For this review, take the finished solid that the model builds, in its own axes (mm). A direction names the side the tool comes from. Coordinates: 2 decimals unless noted, no trailing zeros. Order: outer loops, then holes, each group sorted by start corner. A loop starts at its lowest first (then second) coordinate and runs counter-clockwise, first axis right, second up. Notation, with made-up numbers: M 69,38 L 97,38 A12 cw 97,52 Z; hole C -9,37.5 d7. An arc over 180 degrees is marked long. Use CSV: the item, a comma, the result in double quotes.
```python
from build123d import *

# Parameters (mm, degrees)
SKETCH1_R           = 5
BOSS_EXTRUDE1_DEPTH = 10


with BuildPart() as part:
    # Sketch1 → Boss-Extrude1 (new body)
    with BuildSketch(Plane(origin=(0, 0, 0), x_dir=(1, 0, 0), z_dir=(0, 1, 0))):
        with BuildLine():
            ThreePointArc((7.500789876, 99.718293965), (6.250885533, 99.804440934), (5, 99.874921777))
            Line((5, 99.874921777), (5, 57.735026919))
            ThreePointArc((5, 57.735026919), (0, 52.735026919), (-5, 57.735026919))
            Line((-5, 57.735026919), (-5, 99.874921777))
            ThreePointArc((-5, 99.874921777), (-6.250885533, 99.804440934), (-7.500789876, 99.718293965))
            ThreePointArc((-7.500789876, 99.718293965), (-32.617513459, 56.495190528), (-82.608180857, 56.355021564))
            ThreePointArc((-82.608180857, 56.355021564), (-83.307738492, 55.315646135), (-83.99421946, 54.267587908))
            Line((-83.99421946, 54.267587908), (-47.5, 33.197640478))
            ThreePointArc((-47.5, 33.197640478), (-45.669872981, 26.367513459), (-52.5, 24.537386441))
            Line((-52.5, 24.537386441), (-88.99421946, 45.60733387))
            ThreePointArc((-88.99421946, 45.60733387), (-89.558624026, 44.488794799), (-90.108970734, 43.363272401))
            ThreePointArc((-90.108970734, 43.363272401), (-65.235026919, 0), (-90.108970734, -43.363272401))
            ThreePointArc((-90.108970734, -43.363272401), (-89.558624026, -44.488794799), (-88.99421946, -45.60733387))
            Line((-88.99421946, -45.60733387), (-52.5, -24.537386441))
            ThreePointArc((-52.5, -24.537386441), (-45.669872981, -26.367513459), (-47.5, -33.197640478))
            Line((-47.5, -33.197640478), (-83.99421946, -54.267587908))
            ThreePointArc((-83.99421946, -54.267587908), (-83.307738492, -55.315646135), (-82.608180857, -56.355021564))
            ThreePointArc((-82.608180857, -56.355021564), (-32.617513459, -56.495190528), (-7.500789876, -99.718293965))
            ThreePointArc((-7.500789876, -99.718293965), (-6.250885533, -99.804440934), (-5, -99.874921777))
            Line((-5, -99.874921777), (-5, -57.735026919))
            ThreePointArc((-5, -57.735026919), (0, -52.735026919), (5, -57.735026919))
            Line((5, -57.735026919), (5, -99.874921777))
            ThreePointArc((5, -99.874921777), (6.250885533, -99.804440934), (7.500789876, -99.718293965))
            ThreePointArc((7.500789876, -99.718293965), (32.617513459, -56.495190528), (82.608180857, -56.355021564))
            ThreePointArc((82.608180857, -56.355021564), (83.307738492, -55.315646135), (83.99421946, -54.267587908))
            Line((83.99421946, -54.267587908), (47.5, -33.197640478))
            ThreePointArc((47.5, -33.197640478), (45.669872981, -26.367513459), (52.5, -24.537386441))
            Line((52.5, -24.537386441), (88.99421946, -45.60733387))
            ThreePointArc((88.99421946, -45.60733387), (89.558624026, -44.488794799), (90.108970734, -43.363272401))
            ThreePointArc((90.108970734, -43.363272401), (65.235026919, 0), (90.108970734, 43.363272401))
            ThreePointArc((90.108970734, 43.363272401), (89.558624026, 44.488794799), (88.99421946, 45.60733387))
            Line((88.99421946, 45.60733387), (52.5, 24.537386441))
            ThreePointArc((52.5, 24.537386441), (45.669872981, 26.367513459), (47.5, 33.197640478))
            Line((47.5, 33.197640478), (83.99421946, 54.267587908))
            ThreePointArc((83.99421946, 54.267587908), (83.307738492, 55.315646135), (82.608180857, 56.355021564))
            ThreePointArc((82.608180857, 56.355021564), (32.617513459, 56.495190528), (7.500789876, 99.718293965))
        make_face()
        with Locations(Location((0, 0, 0), (0, 0, 270))):  # turned: the seam where the file's is
            Circle(SKETCH1_R, mode=Mode.SUBTRACT)
    extrude(amount=BOSS_EXTRUDE1_DEPTH)


solid = part.part
```
Item 1: Clearance check with flat-ended pins moving along their axes: pin 1 Ø6 at (y, z) = (6, 42.5) entering from -X; pin 2 Ø3 at (y, z) = (5.5, -44) entering from +X; pin 3 Ø3 at (y, z) = (5, -88) entering from -X; pin 4 Ø2 at (x, y) = (5.5, 6) entering from +Z. State where each tip first meets the part, or that it passes through.
Solutions:
pin 1,"x = -90.11"
pin 2,"x = 90.11"
pin 3,"x = -9.35"
pin 4,"z = 99.87"
Item 2: Add section B-B on z = 0. State the section outline as (x, y) points, and give its area (3 significant figures).
Solutions:
outline,"M -65.24,0 L -5,0 L -5,10 L -65.24,10 Z; M 5,0 L 65.24,0 L 65.24,10 L 5,10 Z"
area,"1,200 mm^2"
Item 3: Add section A-A on x = 0. State the section outline as (y, z) points.
Solutions:
outline,"M 0,-52.74 L 10,-52.74 L 10,-5 L 0,-5 Z; M 0,5 L 10,5 L 10,52.74 L 0,52.74 Z"
Item 4: For faces 1 (the face through (-66, 4.93, -43.88)), 2 (the face through (5, 5, -79)), 3 (the face through (65.24, 4.93, 0.73)), 4 (the face through (5, 5, 79)), list the 3-axis set-ups (+Z, -Z, +X, -X, +Y, -Y) from which the entire face can be reached by the end or side of a thin tool; tool diameter is ignored.
Solutions:
face 1,"+Y, -Y"
face 2,"-Z, +Y, -Y"
face 3,"+X, +Y, -Y"
face 4,"+Z, +Y, -Y"
Item 5: Add section D-D on x = -68.5. State the section outline as (y, z) points (3 decimals), and give its area (3 significant figures).
Solutions:
outline,"M 0,-50.932 L 10,-50.932 L 10,-45.322 L 0,-45.322 Z; M 0,-33.775 L 10,-33.775 L 10,-17.815 L 0,-17.815 Z; M 0,17.815 L 10,17.815 L 10,33.775 L 0,33.775 Z; M 0,45.322 L 10,45.322 L 10,50.932 L 0,50.932 Z"
area,"431 mm^2"
Item 6: Add section C-C on z = 37.5. State the section outline as (x, y) points.
Solutions:
outline,"M -82.04,0 L -74.95,0 L -74.95,10 L -82.04,10 Z; M -54.95,0 L 54.95,0 L 54.95,10 L -54.95,10 Z; M 74.95,0 L 82.04,0 L 82.04,10 L 74.95,10 Z"
Item 7: Draft analysis for pull direction Z (two halves, no side actions). For faces 5 (the face through (31.986, 4.93, 56.866)), 6 (the face through (66, 4.93, 43.88)), 7 (the face through (45.726, 4.93, -26.273)), 8 (the face through (-5, 5, -79)), state which applies: released by +Z, released by -Z, zero draft, split by the parting line, or undercut.
Solutions:
face 5,"released by +Z"
face 6,"undercut"
face 7,"undercut"
face 8,"zero draft"
Item 8: To check wall thickness, follow line 1 along X through (y, z) = (5, 26); line 2 along X through (y, z) = (7.25, 25.5); line 3 along X through (y, z) = (7.75, 55.5). State the ranges of each line that lie inside material, in increasing order. Write a range as [from, to].
Solutions:
line 1,"[-72.49, -55.03], [-45.9, 45.9], [55.03, 72.49]"
line 2,"[-72.19, -54.17], [-46.3, 46.3], [54.17, 72.19]"
line 3,"[-83.19, -81.04], [-34.43, -4.47], [4.47, 34.43], [81.04, 83.19]"
